```python
from build123d import *

# Parameters (mm, degrees)
F0_W     = 25
F0_H     = 24.6772709091
F0_H_2   = 25
F1_DEPTH = 1


with BuildPart() as f1:
    # F0 (on Front) → F1 (new body)
    with BuildSketch(Plane.XZ):
        with Locations((-12.5, 12.3386354545)):
            Rectangle(F0_W, F0_H)
        Polygon((0, 24.6772709091), (0, 0), (25, -0.3227290909), (25, 24.6772709091), align=None)
        with Locations((12.5, 37.1772709091)):
            Rectangle(F0_W, F0_H_2)
        with Locations((37.5, 12.1772709091)):
            Rectangle(F0_W, F0_H_2)
        Polygon((25, -0.3227290909), (0, 0), (0, -25.3227290909), (25, -25.3227290909), align=None)
        Polygon((1.8516593846, 53.4272709091), (0, 49.6772709091), (25, 49.6772709091), (21.8516593846, 53.4272709091), align=None)
        Polygon((-25, 24.6772709091), (0, 24.6772709091), (-3.4180502594, 28.4272709091), (-23.4180502594, 28.4272709091), align=None)
        Polygon((-28.75, 3.0904370546), (-25, 0), (-25, 24.6772709091), (-28.75, 23.0904370546), align=None)
        Polygon((-3.4180502594, -3.75), (0, 0), (-25, 0), (-23.4180502594, -3.75), align=None)
        Polygon((25, -25.3227290909), (0, -25.3227290909), (1.8516593846, -29.0727290909), (21.8516593846, -29.0727290909), align=None)
        Polygon((50, -0.3227290909), (25, -0.3227290909), (26.9035287201, -4.0727290909), (46.9035287201, -4.0727290909), align=None)
        Polygon((50, 24.6772709091), (50, -0.3227290909), (53.75, 3.0904370546), (53.75, 23.0904370546), align=None)
        Polygon((27.1213706583, 28.4272709091), (25, 24.6772709091), (50, 24.6772709091), (47.1213706583, 28.4272709091), align=None)
    extrude(amount=F1_DEPTH)


solid = f1.part
```
Input: part model. Units: mm. Frame: model coordinates. Round coordinates to 2 decimals unless told otherwise and drop trailing zeros. Order: outer loops, then holes, each group sorted by start corner. A loop starts at its lowest first (then second) coordinate and runs counter-clockwise, first axis right, second up. Notation, with made-up numbers: (63.5, 2.25) - (92.5, 2.25) arc R14 ccw to (92.5, 23.25) - close; hole circle Ø10 at (14.25, 6.5). An arc over 180 degrees is marked (long way). One line per question, with ' | ' between items. Start each with the question number.
1) Cut plane D-D, the plane z = -19. Return the cut outline in (x, y), then the cut area to 3 significant figures.
2) Contact query for flat-ended pins moving along their axis: P1, Ø12, axis at x = 32, z = 10.5, coming from the +Y side; P2, Ø0.5, axis at y = -0.5, z = -10, coming from the -X side. Output: stop coordinate, or through.
3) Ray query, probe 1 along X at (y, z) = (-0.05, 27.5); probe 2 along X at (y, z) = (-0.75, -22.5); probe 3 along Z at (x, y) = (45.5, -0.8). Return the intervals inside material, ascending.
4) Pull-direction query (X, two-part tool) for faces 1 (the flat face through (12, 0, 13)), 2 (the flat face through (26.076, -0.493, 26.579)), 3 (the flat face through (0.91, -0.49, -27.17)); classes: +X half, -X half, draft (parallel to the pull), parting line (faces both ways), or undercut.
5) Cut plane B-B, the plane z = 27. Return the cut outline in (x, y), then the cut area to 3 significant figures.
6) Cut plane C-C, the plane x = 31.5. Return the cut outline in (y, z).
7) Cut plane A-A, the plane y = -0.65. Return the cut outline in (x, z), then the cut area to 3 significant figures.
Worked out:
1) outline: (0, -1) - (25, -1) - (25, 0) - (0, 0) - close | area: 25.0 mm^2
2) P1: stops at y = 0 | P2: stops at x = 0
3) probe 1: x = -23.81 to -2.57, 0 to 25, 26.6 to 47.83 | probe 2: x = 0 to 25 | probe 3: z = -4.07 to 28.43
4) face 1: draft | face 2: undercut | face 3: -X half
5) outline: (-24.02, -1) - (-2.12, -1) - (-2.12, 0) - (-24.02, 0) - close; (0, -1) - (25, -1) - (25, 0) - (0, 0) - close; (26.31, -1) - (48.22, -1) - (48.22, 0) - (26.31, 0) - close | area: 68.8 mm^2
6) outline: (-1, -4.07) - (0, -4.07) - (0, 28.43) - (-1, 28.43) - close
7) outline: (-28.75, 3.09) - (-25, 0) - (-23.42, -3.75) - (-3.42, -3.75) - (0, 0) - (0, -25.32) - (1.85, -29.07) - (21.85, -29.07) - (25, -25.32) - (25, -0.32) - (26.9, -4.07) - (46.9, -4.07) - (50, -0.32) - (53.75, 3.09) - (53.75, 23.09) - (50, 24.68) - (47.12, 28.43) - (27.12, 28.43) - (25, 24.68) - (25, 49.68) - (21.85, 53.43) - (1.85, 53.43) - (0, 49.68) - (0, 24.68) - (-3.42, 28.43) - (-23.42, 28.43) - (-25, 24.68) - (-28.75, 23.09) - close | area: 3,790 mm^2
